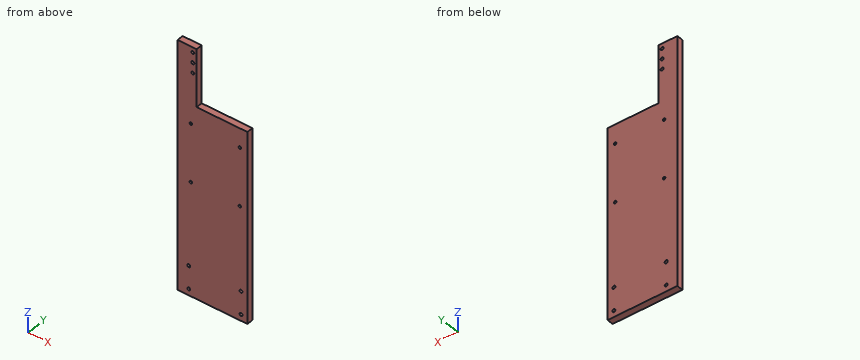
from build123d import *

# Parameters (mm, degrees)
SKETCH1_W           = 69.85
SKETCH1_H           = 247.65
BOSS_EXTRUDE1_DEPTH = 6.35
SKETCH2_W           = 50.8
SKETCH2_H           = 57.404
CUT_EXTRUDE1_DEPTH  = 7.35
SKETCH3_R           = 1.499997
CUT_EXTRUDE2_DEPTH  = 7.35
SKETCH4_R           = 1.499997
CUT_EXTRUDE3_DEPTH  = 7.35
SKETCH5_R           = 1.25
CUT_EXTRUDE4_DEPTH  = 7.35


with BuildPart() as part:
    # Sketch1 → Boss-Extrude1 (new body)
    with BuildSketch(Plane(origin=(0, 0, 0), x_dir=(1, 0, 0), z_dir=(0, 1, 0))):
        with Locations((34.925, 123.825)):
            Rectangle(SKETCH1_W, SKETCH1_H)
    extrude(amount=BOSS_EXTRUDE1_DEPTH)

    # Sketch2 → Cut-Extrude1 (cut, through all)
    with BuildSketch(Plane(origin=(0, 6.35, 0), x_dir=(1, 0, 0), z_dir=(0, 1, 0))):
        with Locations((44.45, 28.702)):
            Rectangle(SKETCH2_W, SKETCH2_H)
    extrude(amount=-CUT_EXTRUDE1_DEPTH, mode=Mode.SUBTRACT)

    # Sketch3 → Cut-Extrude2 (cut, through all)
    with BuildSketch(Plane(origin=(0, 6.35, 0), x_dir=(1, 0, 0), z_dir=(0, 1, 0))):
        with Locations((15.24, 5.08)):
            Circle(SKETCH3_R)
        with Locations((15.24, 25.4)):
            Circle(SKETCH3_R)
        with Locations((15.24, 15.24)):
            Circle(SKETCH3_R)
    extrude(amount=-CUT_EXTRUDE2_DEPTH, mode=Mode.SUBTRACT)

    # Sketch4 → Cut-Extrude3 (cut, through all)
    with BuildSketch(Plane(origin=(0, 6.35, 0), x_dir=(1, 0, 0), z_dir=(0, 1, 0))):
        with Locations((63.5, 241.3)):
            Circle(SKETCH4_R)
        with Locations((63.5, 218.3)):
            Circle(SKETCH4_R)
        with Locations((11.2, 218.3)):
            Circle(SKETCH4_R)
        with Locations((11.2, 241.3)):
            Circle(SKETCH4_R)
    extrude(amount=-CUT_EXTRUDE3_DEPTH, mode=Mode.SUBTRACT)

    # Sketch5 → Cut-Extrude4 (cut, through all)
    with BuildSketch(Plane(origin=(0, 6.35, 0), x_dir=(1, 0, 0), z_dir=(0, 1, 0))):
        with Locations((13.23, 134.454)):
            Circle(SKETCH5_R)
        with Locations((62.23, 134.454)):
            Circle(SKETCH5_R)
        with Locations((62.23, 76.454)):
            Circle(SKETCH5_R)
        with Locations((13.23, 76.454)):
            Circle(SKETCH5_R)
    extrude(amount=-CUT_EXTRUDE4_DEPTH, mode=Mode.SUBTRACT)


solid = part.part
For this review, take the finished solid that the model builds, in its own axes (mm). Give positions to 0.01 mm unless a question says otherwise; leave off trailing zeros. Order: outer loops, then holes, each group sorted by start corner. A loop starts at its lowest first (then second) coordinate and runs counter-clockwise, first axis right, second up. Notation, with made-up numbers: M 21,69 L 57,69 A18 ccw 57,101 Z; hole C 69,72 d8. An arc over 180 degrees is marked long. Answer in a Markdown table with one row per item. Add a question column.
(1) Wall thickness on probe 1 along Z at (x, y) = (11.2, 4.75); probe 2 along X at (y, z) = (2.25, -218.3); probe 3 along Z at (x, y) = (13.23, 2.5): over which ranges is each line inside the solid? List them lowest first. Write a range as [from, to].
(2) Consider section B-B on z = -21. State the section outline as (x, y) points.
(3) Consider section A-A on y = 4.75. Give the number of separate pieces and of enclosed holes in the cut face, and give its area (3 significant figures).
(4) Consider section C-C on x = 50. State the section outline as (y, z) points.
(5) For pin 1 (3 mm diameter, centred on y = 2.5, z = -15.5, fed in from +X), flat-tipped, find the tip position at first contact; note if it passes through.
Evaluation:
| question | item | result |
|---|---|---|
| 1 | probe 1 | z = [-247.65, -242.8], [-239.8, -219.8], [-216.8, 0] |
| 1 | probe 2 | x = [0, 9.7], [12.7, 62], [65, 69.85] |
| 1 | probe 3 | z = [-247.65, -135.7], [-133.2, -77.7], [-75.2, 0] |
| 2 | outline | M 0,0 L 19.05,0 L 19.05,6.35 L 0,6.35 Z |
| 3 | separate pieces | 1 |
| 3 | enclosed holes | 11 |
| 3 | area | 14,300 mm^2 |
| 4 | outline | M 0,-247.65 L 6.35,-247.65 L 6.35,-57.4 L 0,-57.4 Z |
| 5 | pin 1 | stops at x = 19.05 |
